Geometry: final body of the model. Coordinates: model frame, mm. Give positions to 0.01 mm unless a question says otherwise; leave off trailing zeros. Write each loop counter-clockwise with the first axis right and the second up, starting at its lowest first coordinate (ties: lowest second). Pieces come first, ordered by that corner, then holes.
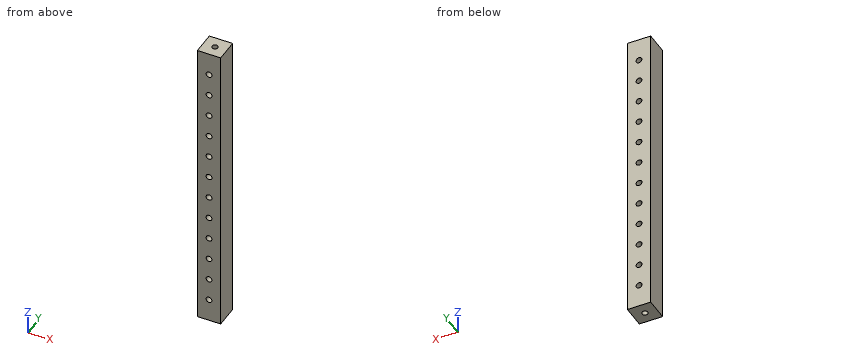
from build123d import *

# Parameters (mm, degrees)
F0_W      = 10
F0_H      = 10
F1_DEPTH  = 130
F3_D      = 2.5
F3_DEPTH  = 10
F5_D      = 2.5
F5_DEPTH  = 10
F7_D      = 2.5
F7_DEPTH  = 10
F9_D      = 2.5
F9_DEPTH  = 10
F11_D     = 2.5
F11_DEPTH = 10
F13_D     = 2.5
F13_DEPTH = 10
F15_D     = 2.5
F15_DEPTH = 10


with BuildPart() as f1:
    # F0 (on Top) → F1 (new body)
    with BuildSketch(Plane.XY):
        with Locations((5, 5)):
            Rectangle(F0_W, F0_H)
    extrude(amount=F1_DEPTH)

    # F3
    with Locations(Plane.XZ):
        with Locations((5, 10), (5, 20), (5, 30)):
            Hole(F3_D / 2, depth=F3_DEPTH)

    # F5
    with Locations(Plane.XZ):
        with Locations((5, 40), (5, 50), (5, 60)):
            Hole(F5_D / 2, depth=F5_DEPTH)

    # F7
    with Locations(Plane.XZ):
        with Locations((5, 80), (5, 90), (5, 100), (5, 110)):
            Hole(F7_D / 2, depth=F7_DEPTH)

    # F9
    with Locations(Plane.XZ):
        with Locations((5, 70)):
            Hole(F9_D / 2, depth=F9_DEPTH)

    # F11
    with Locations(Plane.XZ):
        with Locations((5, 120)):
            Hole(F11_D / 2, depth=F11_DEPTH)

    # F13
    with Locations(Plane.XY.offset(130)):
        with Locations((5, 5)):
            Hole(F13_D / 2, depth=F13_DEPTH)

    # F15
    with Locations(Plane(origin=(0, 0, 0), x_dir=(1, 0, 0), z_dir=(0, 0, -1))):
        with Locations((5, -5)):
            Hole(F15_D / 2, depth=F15_DEPTH)


solid = f1.part
Q1. Ray query, line 1 along X through (y, z) = (3.75, 90); line 2 along X through (y, z) = (1.75, 121). Return the intervals inside material, ascending.
Filled sheet:
line 1: x = 0 to 3.75, 6.25 to 10
line 2: x = 0 to 4.25, 5.75 to 10
Q2. Pin query (flat end, axial travel): P1, Ø2, axis at x = 5, z = 60, coming from the +Y side; P2, Ø2, axis at x = 5, y = 5, coming from the -Z side; P3, Ø1.5, axis at x = 5, y = 5, coming from the -Z side. Return the tip coordinate at first contact, or that it passes through.
Filled sheet:
P1: passes through
P2: stops at z = 10.75
P3: stops at z = 11
Q3. Section B-B on z = 30. Output: boundary loops of the cut face in (x, y), plus the area to 3 significant figures.
Filled sheet:
outline: (0, 0) - (3.75, 0) - (3.75, 10) - (0, 10) - close; (6.25, 0) - (10, 0) - (10, 10) - (6.25, 10) - close
area: 75.0 mm2
Q4. Section A-A on y = 2.5. Count the separate pieces of the cut face and the enclosed holes in it, plus the area to 3 significant figures.
Filled sheet:
separate pieces: 1
enclosed holes: 12
area: 1,240 mm2
